```python
from build123d import *

# Parameters (mm, degrees)
BOSS_EXTRUDE2_DEPTH = 1.5875


with BuildPart() as part:
    # Sketch1 → Boss-Extrude2 (new body)
    with BuildSketch(Plane(origin=(0, 0, 0), x_dir=(1, 0, 0), z_dir=(0, 1, 0))):
        Polygon((-171.45, 76.2), (-44.45, 0), (0, 0), (0, 228.6), (-123.825, 228.6), (-123.825, 158.75), (-155.575, 158.75), (-155.575, 228.6), (-171.45, 228.6), align=None)
        Polygon((0, 228.6), (0, 0), (44.45, 0), (171.45, 76.2), (171.45, 228.6), (155.575, 228.6), (155.575, 158.75), (123.825, 158.75), (123.825, 228.6), align=None)
    extrude(amount=BOSS_EXTRUDE2_DEPTH)


solid = part.part
```
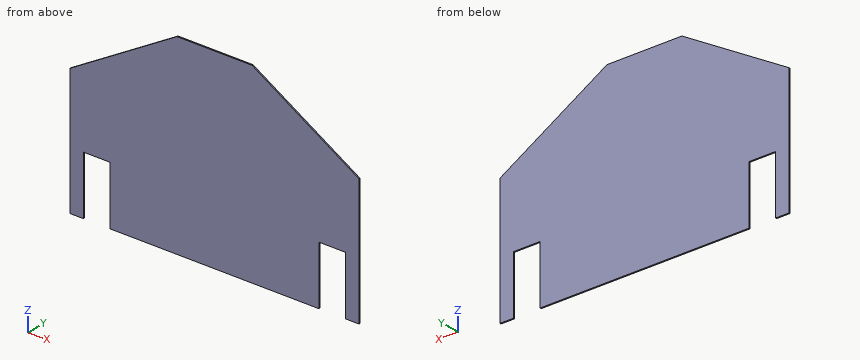
For this review, take the finished solid that the model builds, in its own axes (mm). Coordinates: 2 decimals unless noted, no trailing zeros. Write each loop counter-clockwise with the first axis right and the second up, starting at its lowest first coordinate (ties: lowest second). Pieces come first, ordered by that corner, then holes. Notation, with made-up numbers: (4.25, 71.5) - (58.25, 71.5) arc R32 ccw to (58.25, 100.5) - close; hole circle Ø6 at (52, 0.5). An arc over 180 degrees is marked (long way). Answer in a Markdown table with one row per item. Add a question column.
Q1. For P1, Ø1, axis at x = 97, z = -124.5, coming from the -Y side, flat-tipped, find the tip position at first contact; note if it passes through.
Q2. We need section C-C, the plane x = 140. State the section outline as (y, z) points, and give its area (3 significant figures).
Q3. We need section D-D, the plane x = 58. State the section outline as (y, z) points.
Q4. We need section A-A, the plane z = -174. Count the separate pieces of the cut face and the enclosed holes in it, and give its area (3 significant figures).
Q5. We need section B-B, the plane y = 0.7. State the section outline as (x, z) points (3 decimals).
Q6. For probe 1 along X at (y, z) = (1.4, -174.5) (3 decimals); probe 2 along X at (y, z) = (1.1, -71); probe 3 along X at (y, z) = (0.5, -68), list the stretches that pass through material, from the lowest coordinate up.
Answer list:
| question | item | result |
|---|---|---|
| 1 | P1 | stops at y = 0 |
| 2 | outline | (0, -158.75) - (1.59, -158.75) - (1.59, -57.33) - (0, -57.33) - close |
| 2 | area | 161 mm2 |
| 3 | outline | (0, -228.6) - (1.59, -228.6) - (1.59, -8.13) - (0, -8.13) - close |
| 4 | separate pieces | 3 |
| 4 | enclosed holes | 0 |
| 4 | area | 444 mm2 |
| 5 | outline | (-171.45, -228.6) - (-155.575, -228.6) - (-155.575, -158.75) - (-123.825, -158.75) - (-123.825, -228.6) - (123.825, -228.6) - (123.825, -158.75) - (155.575, -158.75) - (155.575, -228.6) - (171.45, -228.6) - (171.45, -76.2) - (44.45, 0) - (-44.45, 0) - (-171.45, -76.2) - close |
| 6 | probe 1 | x = -171.45 to -155.575, -123.825 to 123.825, 155.575 to 171.45 |
| 6 | probe 2 | x = -162.78 to 162.78 |
| 6 | probe 3 | x = -157.78 to 157.78 |
